Here's how the part is built. I have some questions about the finished solid (model axes, mm). Coordinates: 2 decimals unless noted, no trailing zeros. Write each loop counter-clockwise with the first axis right and the second up, starting at its lowest first coordinate (ties: lowest second). Pieces come first, ordered by that corner, then holes. Notation, with made-up numbers: M -5,87.25 L 35,87.25 A17 cw 35,95.25 Z; hole C 35.25,-21 d6. An arc over 180 degrees is marked long. Write each question's results on one line, items separated by ' | '. Start each with the question number.
from build123d import *

# Parameters (mm, degrees)
F0_W     = 1879.6
F0_H     = 650.875
F1_DEPTH = 26.9875
F2_R     = 5.08
F3_R     = 27.559
F4_DEPTH = 1052.5125
F4_TAPER = 0.25
F5_SCALE = 0.05


with BuildPart() as f1:
    # F0 (on Top) → F1 (new body)
    with BuildSketch(Plane.XY):
        Rectangle(F0_W, F0_H)
    extrude(amount=F1_DEPTH)

    # F2
    f2_edges = [f1.edges().sort_by_distance(p)[0] for p in [
        (-939.8, 325.4375, 13.49375),
        (-939.8, -325.4375, 13.49375),
        (939.8, -325.4375, 13.49375),
        (0, -325.4375, 0),
        (0, -325.4375, 26.9875),
        (-939.8, 0, 0),
        (-939.8, 0, 26.9875),
        (939.8, 325.4375, 13.49375),
        (0, 325.4375, 0),
        (0, 325.4375, 26.9875),
        (939.8, 0, 0),
        (939.8, 0, 26.9875),
    ]]
    fillet(f2_edges, radius=F2_R)

    # F3 (on face) → F4 (join)
    with BuildSketch(Plane(origin=(0, 0, 0), x_dir=(1, 0, 0), z_dir=(0, 0, -1))):
        with Locations((-860.425, 246.0625)):
            Circle(F3_R)
        with Locations((-860.425, -246.0625)):
            Circle(F3_R)
        with Locations((860.425, 246.0625)):
            Circle(F3_R)
        with Locations((860.425, -246.0625)):
            Circle(F3_R)
    extrude(amount=F4_DEPTH, taper=F4_TAPER)


with BuildPart() as f1_1:
    # F5: moved
    add(f1.part.scale(F5_SCALE))


solid = f1_1.part
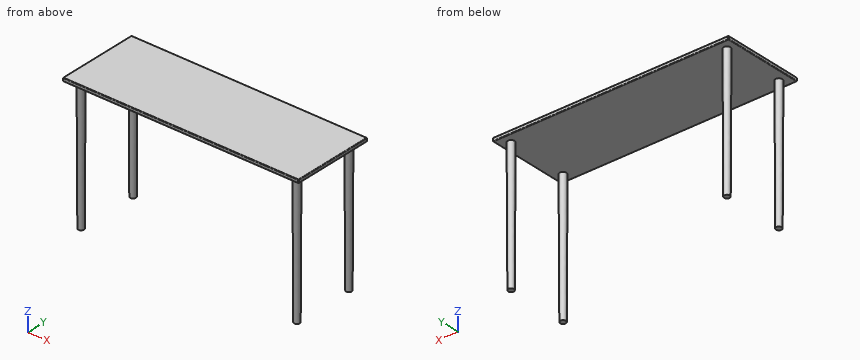
1) For pin 1 Ø3 at (x, y) = (25, 1.5) entering from -Z; pin 2 Ø4 at (y, z) = (12, -14) entering from +X, each with a flat end and sliding along its axis, tell me the tip position at first contact or that it passes through.
2) Please list where these lines run through material, in increasing order: line 1 (X direction, y = -12, z = -11.5); line 2 (Z direction, x = 23, y = -14); line 3 (X direction, y = -11.5, z = -23). Write a range as [from, to].
3) I want a section at A-A, the plane x = 3.5. Write out the boundary of the cut face in (y, z), then the cut area to 3 significant figures.
4) I want a section at D-D, the plane z = -39.5. Write out the boundary of the cut face in (x, y).
5) I want a section at B-B, the plane y = -8. Write out the boundary of the cut face in (x, z), then the cut area to 3 significant figures.
6) I want a section at C-C, the plane z = -19. Write out the boundary of the cut face in (x, y).
Output:
1) pin 1: stops at z = 0 | pin 2: stops at x = 44.35
2) line 1: x = [-44.31, -41.73], [41.73, 44.31] | line 2: z = [0, 1.35] | line 3: x = [-44.01, -42.03], [42.03, 44.01]
3) outline: M -16.27,0.25 A0.25 ccw -16.02,0 L 16.02,0 A0.25 ccw 16.27,0.25 L 16.27,1.1 A0.25 ccw 16.02,1.35 L -16.02,1.35 A0.25 ccw -16.27,1.1 Z | area: 43.9 mm2
4) outline: C -43.02,-12.3 d2.41; C -43.02,12.3 d2.41; C 43.02,-12.3 d2.41; C 43.02,12.3 d2.41
5) outline: M -46.99,0.25 A0.25 ccw -46.74,0 L 46.74,0 A0.25 ccw 46.99,0.25 L 46.99,1.1 A0.25 ccw 46.74,1.35 L -46.74,1.35 A0.25 ccw -46.99,1.1 Z | area: 127 mm2
6) outline: C -43.02,-12.3 d2.59; C -43.02,12.3 d2.59; C 43.02,-12.3 d2.59; C 43.02,12.3 d2.59
